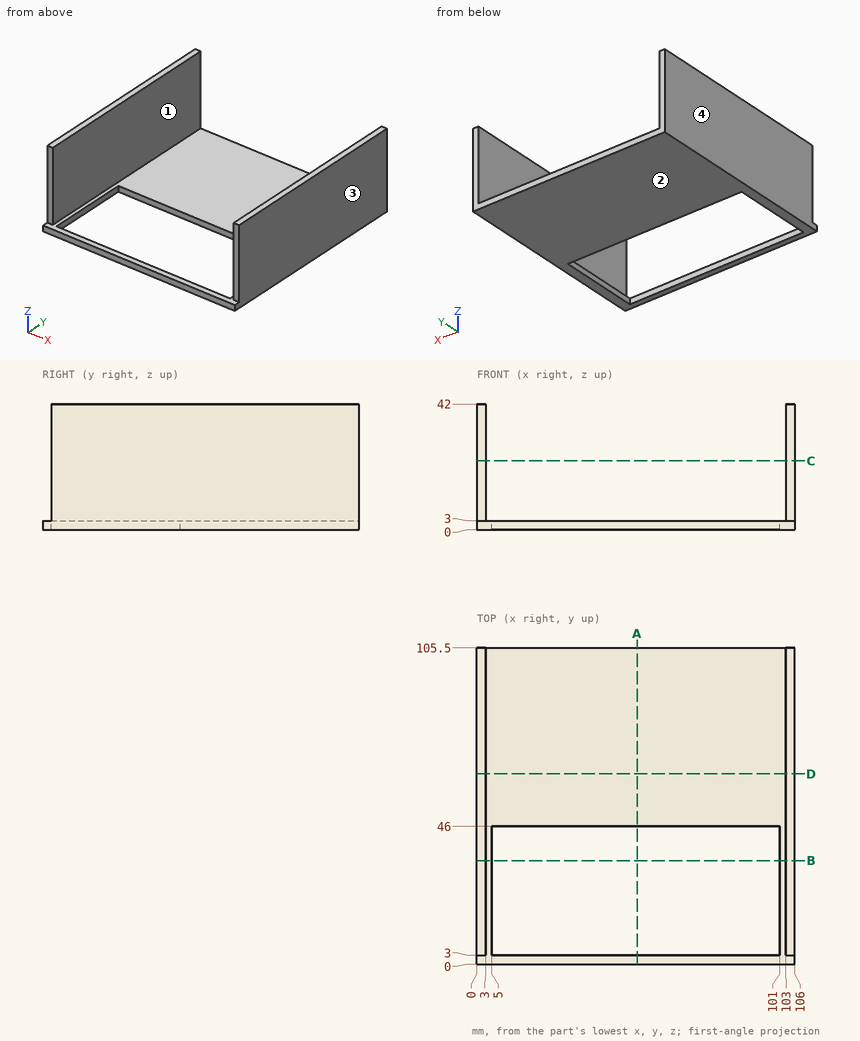
Can you work these out from the drawing? Everything is in mm from the part's minimum corner. Give positions to 0.01 mm unless a question says otherwise; leave off trailing zeros. Order: outer loops, then holes, each group sorted by start corner. A loop starts at its lowest first (then second) coordinate and runs counter-clockwise, first axis right, second up. Notation, with made-up numbers: M 51,-34.5 L 86,-34.5 A15 ccw 86,-16.5 Z; hole C 35.5,-30 d10. An arc over 180 degrees is marked long. One line per question, with ' | ' between items.
1. I want a section at C-C (z = 23). List the corners of the cut face in (x, y) for me, and give its area (3 significant figures).
Results:
outline: M 0,3 L 3,3 L 3,105.5 L 0,105.5 Z; M 103,3 L 106,3 L 106,105.5 L 103,105.5 Z | area: 615 mm²
2. I'm going to push flat-ended pins straight in: pin 1 (2 mm diameter, centred on x = 75.5, y = 51.5, fed in from +Z); pin 2 (2.5 mm diameter, centred on x = 104, z = 17, fed in from -Y). Where does each tip first touch, or does it pass through?
Results:
pin 1: z = 3 | pin 2: y = 3
3. I want a section at D-D (y = 63.5). List the corners of the cut face in (x, z) for me, and give its area (3 significant figures).
Results:
outline: M 0,0 L 106,0 L 106,42 L 103,42 L 103,3 L 3,3 L 3,42 L 0,42 Z | area: 552 mm²
4. I want a section at B-B (y = 34.5). List the corners of the cut face in (x, z) for me, and give its area (3 significant figures).
Results:
outline: M 0,0 L 5,0 L 5,3 L 3,3 L 3,42 L 0,42 Z; M 101,0 L 106,0 L 106,42 L 103,42 L 103,3 L 101,3 Z | area: 264 mm²
5. We'd pull the mould along X, two halves only. Please class the marked faces 1, 2, 3 and 4: +X half, -X half, draft (parallel to the pull), parting line (faces both ways), or undercut.
Results:
face 1: undercut | face 2: draft | face 3: +X half | face 4: -X half
6. If I drill on line 1 (X direction, y = 87, z = 24.5); line 2 (Z direction, x = 95.5, y = 59), over which ranges is the centre line in solid material (lowest first)?
Results:
line 1: 0 to 3, 103 to 106 | line 2: 0 to 3
7. I want a section at A-A (x = 53.5). List the corners of the cut face in (y, z) for me, and give its area (4 significant figures).
Results:
outline: M 0,0 L 3,0 L 3,3 L 0,3 Z; M 46,0 L 105.5,0 L 105.5,3 L 46,3 Z | area: 187.5 mm²
